```python
from build123d import *

# Parameters (mm, degrees)
SKETCH1_W           = 16.51
SKETCH1_H           = 16.59
BOSS_EXTRUDE1_DEPTH = 1.52
SKETCH2_W           = 1
SKETCH2_H           = 16.59
BOSS_EXTRUDE2_DEPTH = 7.37


with BuildPart() as part:
    # Sketch1 → Boss-Extrude1 (new body)
    with BuildSketch(Plane(origin=(0, 0, 0), x_dir=(1, 0, 0), z_dir=(0, 1, 0))):
        with Locations((8.255, 8.295)):
            Rectangle(SKETCH1_W, SKETCH1_H)
    extrude(amount=BOSS_EXTRUDE1_DEPTH)

    # Sketch2 → Boss-Extrude2 (add)
    with BuildSketch(Plane(origin=(0, 1.52, 0), x_dir=(1, 0, 0), z_dir=(0, 1, 0))):
        with Locations((0.5, 8.295)):
            Rectangle(SKETCH2_W, SKETCH2_H)
        with Locations((2.715714286, 8.295)):
            Rectangle(SKETCH2_W, SKETCH2_H)
        with Locations((4.931428571, 8.295)):
            Rectangle(SKETCH2_W, SKETCH2_H)
        with Locations((7.147142857, 8.295)):
            Rectangle(SKETCH2_W, SKETCH2_H)
        with Locations((9.362857143, 8.295)):
            Rectangle(SKETCH2_W, SKETCH2_H)
        with Locations((11.578571429, 8.295)):
            Rectangle(SKETCH2_W, SKETCH2_H)
        with Locations((13.794285714, 8.295)):
            Rectangle(SKETCH2_W, SKETCH2_H)
        with Locations((16.01, 8.295)):
            Rectangle(SKETCH2_W, SKETCH2_H)
    extrude(amount=BOSS_EXTRUDE2_DEPTH)


solid = part.part
```
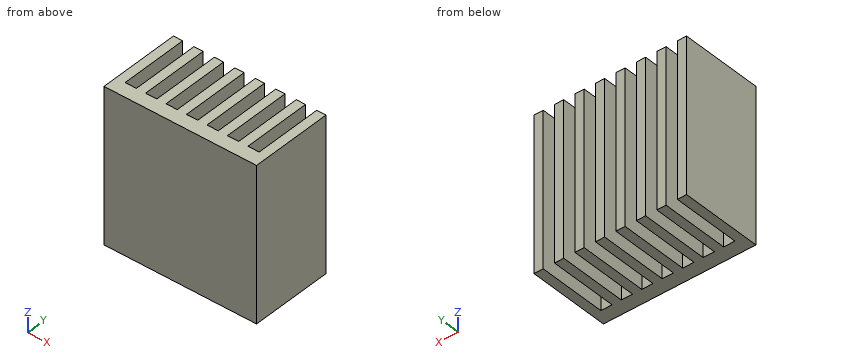
Here's how the part is built. I have some questions about the finished solid (model axes, mm). Coordinates: 2 decimals unless noted, no trailing zeros. Loops run counter-clockwise (first coordinate to the right, second up) from the corner with the lowest first, then second, coordinate; pieces in that order, holes last. Notation, with made-up numbers: (1, 0) - (14, 0) arc R29 cw to (14, 38) - close; hole circle Ø2 at (81.5, -13). An arc over 180 degrees is marked (long way). Answer as CSV lines item,"result".
Q1. If we section it at A-A, the plane y = 7: Give the number of separate pieces and of enclosed holes in the cut face, and give its area (3 significant figures).
Response:
separate pieces,"8"
enclosed holes,"0"
area,"133 mm2"
Q2. For pin 1 (1 mm diameter, centred on x = 10.5, z = -11, fed in from +Y), with a flat end and sliding along its axis, tell me the tip position at first contact or that it passes through.
Response:
pin 1,"y = 1.52"
Q3. If we section it at C-C, the plane x = 3.5: Write out the boundary of the cut face in (y, z).
Response:
outline,"(0, -16.59) - (1.52, -16.59) - (1.52, 0) - (0, 0) - close"
Q4. If I drill on L1, parallel to Y at x = 10, z = -14.75, over which ranges is the centre line in solid material (lowest first)? Write a range as [from, to].
Response:
L1,"[0, 1.52]"
